Input: part model. Units: mm. Frame: model coordinates. Face numbers are marked on the shaded views. A direction names the side the tool comes from. Round coordinates to 2 decimals unless told otherwise and drop trailing zeros. Order: outer loops, then holes, each group sorted by start corner. A loop starts at its lowest first (then second) coordinate and runs counter-clockwise, first axis right, second up. Notation, with made-up numbers: (2, 38) -> (54, 38) arc R32 cw to (54, 75) -> close; hole circle Ø4 at (65, -26). An arc over 180 degrees is marked (long way). Use a Markdown table: item, result.
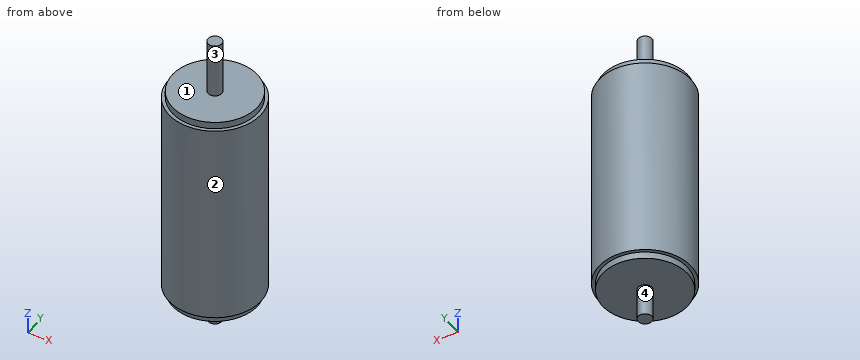
from build123d import *

# Parameters (mm, degrees)
SKETCH1_R           = 100
BOSS_EXTRUDE1_DEPTH = 450
SKETCH2_R           = 92.5
BOSS_EXTRUDE2_DEPTH = 15
SKETCH3_R           = 15
BOSS_EXTRUDE3_DEPTH = 70
BOSS_EXTRUDE4_START = 120
SKETCH4_R           = 15
BOSS_EXTRUDE4_DEPTH = 120
SKETCH5_R           = 1
CUT_EXTRUDE1_DEPTH  = 3


with BuildPart() as part:
    # Sketch1 → Boss-Extrude1 (new body)
    with BuildSketch(Plane.XY):
        Circle(SKETCH1_R)
    extrude(amount=BOSS_EXTRUDE1_DEPTH)

    # Sketch2 → Boss-Extrude2 (add)
    with BuildSketch(Plane(origin=(0, 0, 0), x_dir=(-1, 0, 0), z_dir=(0, 0, -1))):
        Circle(SKETCH2_R)
    boss_extrude2 = extrude(amount=BOSS_EXTRUDE2_DEPTH)

    # Sketch3 → Boss-Extrude3 (add)
    with BuildSketch(Plane(origin=(0, 0, -15), x_dir=(-1, 0, 0), z_dir=(0, 0, -1))):
        Circle(SKETCH3_R)
    extrude(amount=BOSS_EXTRUDE3_DEPTH)

    # Mirror1: Boss-Extrude2 across plane
    add(boss_extrude2.mirror(Plane(origin=(0, 0, 225), x_dir=(1, 0, 0), z_dir=(0, 0, -1))))

    # Sketch4 → Boss-Extrude4 (add)
    with BuildSketch(Plane.XY.offset(465).offset(BOSS_EXTRUDE4_START)):
        with Locations(Location((0, 0, 0), (0, 0, 180))):
            Circle(SKETCH4_R)
    extrude(amount=-BOSS_EXTRUDE4_DEPTH)

    # Sketch5 → Cut-Extrude1 (cut)
    with BuildSketch(Plane(origin=(76.297187213, 64.643168421, 0), x_dir=(0, 0, -1), z_dir=(0.7629718721254075, 0.646431684206035, 0))):
        with Locations(Location((-15, 0, 0), (0, 0, 90))):
            Circle(SKETCH5_R)
    extrude(amount=-CUT_EXTRUDE1_DEPTH, mode=Mode.SUBTRACT)


solid = part.part
1) Line query: L1, parallel to Z at x = -15, y = -92; L2, parallel to Z at x = -38.5, y = 82; L3, parallel to X at y = 4, z = 139. Output: solid intervals per line, ascending. Write a range as [from, to].
Results found:
| item | result |
|---|---|
| L1 | z = [0, 450] |
| L2 | z = [-15, 465] |
| L3 | x = [-99.92, 99.92] |
2) Pull-direction query (X, two-part tool) for the marked faces 1 and 2; classes: +X half, -X half, draft (parallel to the pull), parting line (faces both ways), or undercut.
Results found:
| item | result |
|---|---|
| face 1 | draft |
| face 2 | parting line |
3) Set-up query: the marked faces 3 and 4. Return all of +Z, -Z, +X, -X, +Y, -Y with unobstructed straight access to the full face (end or side cutting, diameter ignored); none if empty.
Results found:
| item | result |
|---|---|
| face 3 | +Z |
| face 4 | -Z |
4) Cut plane D-D on x = -69. Return loops of the section in (y, z).
Results found:
| item | result |
|---|---|
| outline | (-72.38, 0) -> (-61.61, 0) -> (-61.61, -15) -> (61.61, -15) -> (61.61, 0) -> (72.38, 0) -> (72.38, 450) -> (61.61, 450) -> (61.61, 465) -> (-61.61, 465) -> (-61.61, 450) -> (-72.38, 450) -> close |
5) Cut plane C-C on z = 517. Return loops of the section in (x, y), and give its area (3 significant figures).
Results found:
| item | result |
|---|---|
| outline | circle Ø30 at (0, 0) |
| area | 707 mm² |
6) Pin query (flat end, axial travel): pin 1 Ø6 at (x, z) = (27, 175.5) entering from +Y; pin 2 Ø1 at (x, y) = (8, -47) entering from -Z; pin 3 Ø8 at (x, y) = (-26, 43.5) entering from +Z. Return the tip coordinate at first contact, or that it passes through.
Results found:
| item | result |
|---|---|
| pin 1 | stops at y = 97.08 |
| pin 2 | stops at z = -15 |
| pin 3 | stops at z = 465 |
7) Cut plane A-A on y = 0. Return loops of the section in (x, z).
Results found:
| item | result |
|---|---|
| outline | (-100, 0) -> (-92.5, 0) -> (-92.5, -15) -> (-15, -15) -> (-15, -85) -> (15, -85) -> (15, -15) -> (92.5, -15) -> (92.5, 0) -> (100, 0) -> (100, 450) -> (92.5, 450) -> (92.5, 465) -> (15, 465) -> (15, 585) -> (-15, 585) -> (-15, 465) -> (-92.5, 465) -> (-92.5, 450) -> (-100, 450) -> close |
